```python
from build123d import *

# Parameters (mm, degrees)
SKETCH3_W           = 2
SKETCH3_H           = 8.955152332
BOSS_EXTRUDE1_DEPTH = 20
SKETCH4_W           = 2
SKETCH4_H           = 8
BOSS_EXTRUDE2_DEPTH = 19
FILLET1_R           = 2
BOSS_EXTRUDE4_START = -0.065389
SKETCH6_W           = 1.410615846
SKETCH6_H           = 2.020756053
BOSS_EXTRUDE4_DEPTH = 0.065389
BOSS_EXTRUDE5_REACH = 20
SKETCH7_W           = 0.410615846
SKETCH7_H           = 2.003452902


with BuildPart() as part:
    # Sketch2 → Revolve2 (revolve)
    with BuildSketch(Plane.XY):
        Polygon((100, 3), (100, 0), (-100, 0), (-100, 3), (-107, 3), (-107.528980942, 0), (-117.528980942, 0), (-118.410615846, 5), (-122.410615846, 5), (-122.410615846, -5), (122.410615846, -5), (122.410615846, 5), (118.410615846, 5), (117.528980942, 0), (107.528980942, 0), (107, 3), align=None)
    revolve(axis=Axis((-122.410615846, -5, 0), (1, 0, 0)))

    # Sketch3 → Boss-Extrude1 (add)
    with BuildSketch(Plane(origin=(122.410615846, 0, 0), x_dir=(0, 0, -1), z_dir=(1, 0, 0))):
        with Locations((0, -1.477576166)):
            Rectangle(SKETCH3_W, SKETCH3_H)
    extrude(amount=-BOSS_EXTRUDE1_DEPTH)

    # Sketch4 → Boss-Extrude2 (add)
    with BuildSketch(Plane.ZY.offset(122.410615846)):
        with Locations((0, -1)):
            Rectangle(SKETCH4_W, SKETCH4_H)
    extrude(amount=-BOSS_EXTRUDE2_DEPTH)

    # Fillet1
    fillet1_edges = [part.edges().sort_by_distance(p)[0] for p in [
        (-122.410615846, -15, 0),
        (-100, -13, 0),
        (100, -13, 0),
        (122.410615846, -15, 0),
    ]]
    fillet(fillet1_edges, radius=FILLET1_R)

    # Sketch6 → Boss-Extrude4 (add)
    with BuildSketch(Plane(origin=(0, 3, 0), x_dir=(1, 0, 0), z_dir=(0, 1, 0)).offset(BOSS_EXTRUDE4_START)):
        with Locations((-102.705307923, -0.010378027)):
            Rectangle(SKETCH6_W, SKETCH6_H)
    extrude(amount=BOSS_EXTRUDE4_DEPTH)

    # Sketch7 → Boss-Extrude5 (add, up to next)
    with BuildSketch(Plane(origin=(0, 3, 0), x_dir=(1, 0, 0), z_dir=(0, 1, 0)), mode=Mode.PRIVATE) as boss_extrude5_sk1:
        with Locations((102.205307923, -0.001726451)):
            Rectangle(SKETCH7_W, SKETCH7_H)
    boss_extrude5_tool1 = extrude(boss_extrude5_sk1.sketch, amount=-BOSS_EXTRUDE5_REACH, mode=Mode.PRIVATE) - part.part
    add(boss_extrude5_tool1.solids().sort_by_distance((102.205308, 3, 0.001726))[0])
    add(boss_extrude5_tool1.solids().sort_by_distance((102.205308, 3, 0.001726))[1])


solid = part.part
```
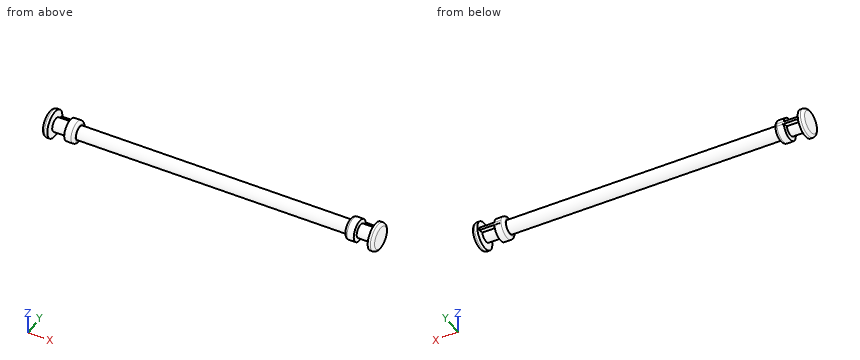
Geometry check sheet. Reference: the model listing, model coordinates, mm. Round coordinates to 2 decimals unless told otherwise and drop trailing zeros. Order: outer loops, then holes, each group sorted by start corner. A loop starts at its lowest first (then second) coordinate and runs counter-clockwise, first axis right, second up. Notation, with made-up numbers: (-38.5, 82) - (-4.5, 82) arc R15 cw to (-4.5, 106) - close; hole circle Ø8 at (-20, -23.5). An arc over 180 degrees is marked (long way). Use a Markdown table: item, result. Add a question column.
1) Thickness scan on line 1 along X through (y, z) = (-2.5, 6.75); line 2 along X through (y, z) = (-10.75, 2.5); line 3 along X through (y, z) = (-7.25, -8). Record the ranges inside material, lowest first.
2) Section check A-A (x = -65.5). Record the cut outline in (y, z).
3) Gauge pin test, flat ends, axial feed: P1, Ø1.6, axis at x = 107, z = 0.5, coming from the +Y side; P2, Ø5, axis at x = -56.5, z = 5.5, coming from the -Y side; P3, Ø5, axis at x = 96, y = 2, coming from the +Z side. Record the tip position at first contact, or that the pin passes through.
Established:
| question | item | result |
|---|---|---|
| 1 | line 1 | -122.41 to -117.92, -107.14 to -100.4, 100.4 to 107.14, 117.92 to 122.41 |
| 1 | line 2 | -122.41 to -117.75, -107.31 to -100.02, 100.02 to 107.31, 117.75 to 122.41 |
| 1 | line 3 | -122.39 to -118.11, 118.11 to 122.39 |
| 2 | outline | circle Ø10 at (-5, 0) |
| 3 | P1 | y = 3 |
| 3 | P2 | y = -9 |
| 3 | P3 | z = 2.18 |
